Read the model definition and answer for the solid it produces. Units are mm, in the model's axes. A direction names the side the tool comes from. Coordinates: 2 decimals unless noted, no trailing zeros. Write each loop counter-clockwise with the first axis right and the second up, starting at its lowest first coordinate (ties: lowest second). Pieces come first, ordered by that corner, then holes. Notation, with made-up numbers: (-30.75, -2) -> (17.25, -2) arc R26 cw to (17.25, 36) -> close; hole circle Ø3 at (8, 11). An arc over 180 degrees is marked (long way). Return JSON: item names as keys, results as strings.
Autodesk Inventor part; units mm, degrees
ref_plane "YZ Plane" through (0, 0, 0) normal (1, 0, 0) x (0, 1, 0)
ref_plane "XZ Plane" through (0, 0, 0) normal (0, 1, 0) x (-1, 0, 0)
ref_plane "XY Plane" through (0, 0, 0) normal (0, 0, 1) x (1, 0, 0)
sketch "Skizze1" plane through (0, 0, 0) normal (0, 0, 1) x (1, 0, 0)
  line L0 (0, 0) -> (80, 0)
  line L1 (80, 0) -> (80, 65)
  line L2 (80, 65) -> (0, 65)
  line L3 (0, 65) -> (0, 0)
  dimension "d0" = 80
  dimension "d1" = 65
extrude "Extrusion2" add sketch "Skizze1" along normal blind 3
sketch "Skizze5" plane through (0, 0, 0) normal (0, -1, 0) x (1, 0, 0)
  line L0 (0, 0) -> (0, 3)
  line L1 (8.5, 8) -> (16.5, 8)
  line L2 (16.5, 8) -> (16.5, 0)
  line L3 (16.5, 0) -> (8.5, 0)
  line L4 (8.5, 0) -> (8.5, 8)
  line L5 (63.5, 8) -> (71.5, 8)
  line L6 (71.5, 8) -> (71.5, 0)
  line L7 (71.5, 0) -> (63.5, 0)
  line L8 (63.5, 0) -> (63.5, 8)
  line L9 (0, 0) -> (80, 0)
  dimension "d105" = 8
  dimension "d108" = 63
  dimension "d109" = 8.5
  dimension "d112" = 8
extrude "Extrusion5" add sketch "Skizze5" along normal blind 20
chamfer "Fase3" distance 9 angle 45 1 edges at (16.5, 0, 1.5)
chamfer "Fase4" distance 9 angle 45 1 edges at (63.5, 0, 1.5)
chamfer "Fase5" distance 3 angle 45 1 edges at (63.5, -4.5, 3)
chamfer "Fase6" distance 3 angle 45 1 edges at (16.5, -4.5, 3)
fillet "Rundung17" radius 4 2 edges at (0, 65, 1.5) (80, 65, 1.5)
sketch "Skizze13" plane through (0, 0, 3) normal (0, 0, 1) x (1, 0, 0)
  line L0 (10, 10) -> (70, 10)
  line L1 (70, 10) -> (70, 0)
  line L2 (70, 0) -> (10, 0)
  line L3 (10, 0) -> (10, 10)
  line L4 (0, 0) -> (8.5, 0)
  line L5 (80, 0) -> (80, 61)
  dimension "d0" = 80
  dimension "d257" = 60
  dimension "d258" = 10
  dimension "d259" = 10
extrude "Extrusion13" add sketch "Skizze13" along normal blind 1
sketch "Skizze15" plane through (0, 0, 4) normal (0, 0, 1) x (1, 0, 0)
  line L0 (10, 2) -> (50, 2)
  line L1 (50, 2) -> (50, 0)
  line L2 (50, 0) -> (10, 0)
  line L3 (10, 0) -> (10, 2)
  line L4 (0, 61) -> (0, 0)
  line L5 (0, 0) -> (8.5, 0)
  dimension "d189" = 40
  dimension "d190" = 2
  dimension "d191" = 10
extrude "Extrusion15" add sketch "Skizze15" along normal blind 2
fillet "Rundung19" radius 1 1 edges at (50, 1, 6)
chamfer "Fase13" distance 2.9999 angle 40 1 edges at (75.75, 0, 0) measured on face at (77.1667, 0, 2)
chamfer "Fase14" distance 2.9999 angle 40 1 edges at (4.25, 0, 0) measured on face at (2.8333, 0, 1)
hole "Bohrung5" at (5, 5, 3) direction (0, 0, -1) diameter 5 end through all
hole "Bohrung6" at (75, 5, 3) direction (0, 0, -1) diameter 5 end through all
hole "Bohrung7" at (4.35, 20, 3) direction (0, 0, -1) diameter 3 end through all
hole "Bohrung8" at (4.35, 50, 3) direction (0, 0, -1) diameter 3 end through all
hole "Bohrung9" at (75.65, 20, 3) direction (0, 0, -1) diameter 3 end through all
hole "Bohrung10" at (75.65, 50, 3) direction (0, 0, -1) diameter 3 end through all
chamfer "Fase16" distance 2 angle 45 1 edges at (65.75, 0, 4)
properties part number "Grundplatte_zerlegt"
1. The part is cut by section B-B (z = 1.75). Determine the outline of the cut face in (x, y).
Taken from the geometry:
{"outline": "(0, 1.05) -> (8.5, 1.05) -> (8.5, -20) -> (16.5, -20) -> (16.5, -9) -> (25.5, 0) -> (54.5, 0) -> (63.5, -9) -> (63.5, -20) -> (71.5, -20) -> (71.5, 1.05) -> (80, 1.05) -> (80, 61) arc R4 ccw to (76, 65) -> (4, 65) arc R4 ccw to (0, 61) -> close; hole circle Ø5 at (5, 5); hole circle Ø3 at (4.35, 20); hole circle Ø3 at (4.35, 50); hole circle Ø5 at (75, 5); hole circle Ø3 at (75.65, 20); hole circle Ø3 at (75.65, 50)"}
2. The part is cut by section C-C (y = 5). Determine the outline of the cut face in (x, z), then the cut area to 3 significant figures.
Taken from the geometry:
{"outline": "(0, 0) -> (2.5, 0) -> (2.5, 3) -> (0, 3) -> close; (7.5, 0) -> (72.5, 0) -> (72.5, 3) -> (70, 3) -> (70, 4) -> (10, 4) -> (10, 3) -> (7.5, 3) -> close; (77.5, 0) -> (80, 0) -> (80, 3) -> (77.5, 3) -> close", "area": "270 mm2"}
3. The part is cut by section A-A (y = 50). Determine the outline of the cut face in (x, z), then the cut area to 3 significant figures.
Taken from the geometry:
{"outline": "(0, 0) -> (2.85, 0) -> (2.85, 3) -> (0, 3) -> close; (5.85, 0) -> (74.15, 0) -> (74.15, 3) -> (5.85, 3) -> close; (77.15, 0) -> (80, 0) -> (80, 3) -> (77.15, 3) -> close", "area": "222 mm2"}
4. Flat-ended cylindrical pins translate along their axes: pin 1 Ø19.5 at (x, y) = (36, 22) entering from +Z; pin 2 Ø2.5 at (x, y) = (4.35, 20) entering from +Z; pin 3 Ø4 at (y, z) = (-13.5, 3.5) entering from +X; pin 4 Ø2.5 at (y, z) = (5, 5) entering from -X. Find the tip coordinate at first contact, or state that the pin passes through.
Taken from the geometry:
{"pin 1": "stops at z = 3", "pin 2": "passes through", "pin 3": "stops at x = 71.5", "pin 4": "stops at x = 10"}
5. A tool of negligible diameter and unlimited length cuts with its end or side. For faces 4 (the face through (75.81, 1.276, 1.479)), 5 (the face through (60.1, -5.6, 1.7)), 6 (the face through (18, -3.4, 4.5)), from which of +Z, -Z, +X, -X, +Y, -Y can it reach the whole face along a straight path? Write none if from no direction.
Taken from the geometry:
{"face 4": "-Z, +X, -Y", "face 5": "+Z, -Z, -Y", "face 6": "+Z, -Y"}
6. The part is cut by section D-D (y = 30.5). Determine the outline of the cut face in (x, z).
Taken from the geometry:
{"outline": "(0, 0) -> (80, 0) -> (80, 3) -> (0, 3) -> close"}
7. For a pull along Y with two mould halves and no side action, classify faces 1 (the face through (4.31, 1.276, 1.479)), 2 (the face through (76.56, 51.19, 1.48)), 3 (the face through (41, 65, 1)) as +Y half, -Y half, draft (parallel to the pull), parting line (faces both ways), or undercut.
Taken from the geometry:
{"face 1": "-Y half", "face 2": "undercut", "face 3": "+Y half"}
8. Consider L1, parallel to X at y = 20, z = 1.6; L2, parallel to X at y = 5, z = 0.9; L3, parallel to Y at x = 75.65, z = 1.75. Determine where each line is inside the solid, lowest interval first.
Taken from the geometry:
{"L1": "x = 0 to 2.85, 5.85 to 74.15, 77.15 to 80", "L2": "x = 0 to 2.5, 7.5 to 72.5, 77.5 to 80", "L3": "y = 1.05 to 2.59, 7.41 to 18.5, 21.5 to 48.5, 51.5 to 65"}
